```python
from build123d import *

# Parameters (mm, degrees)
SKETCH1_W           = 25.4
SKETCH1_H           = 25.4
BOSS_EXTRUDE1_DEPTH = 63.5
SHELL1_T            = -3.175
SKETCH2_R           = 2.4892
CUT_EXTRUDE1_DEPTH  = 63.5
SKETCH3_R           = 2.53492
CUT_EXTRUDE2_DEPTH  = 63.5


with BuildPart() as part:
    # Sketch1 → Boss-Extrude1 (new body)
    with BuildSketch(Plane.XY):
        with Locations((12.7, 12.7)):
            Rectangle(SKETCH1_W, SKETCH1_H)
    extrude(amount=BOSS_EXTRUDE1_DEPTH)

    # Shell1
    shell1_openings = [part.faces().sort_by_distance(p)[0] for p in [
        (12.7, 12.7, 63.5),
        (12.7, 12.7, 0),
    ]]
    offset(amount=SHELL1_T, openings=shell1_openings, kind=Kind.INTERSECTION)

    # Sketch2 → Cut-Extrude1 (cut)
    with BuildSketch(Plane(origin=(0, 25.4, 0), x_dir=(1, 0, 0), z_dir=(0, 1, 0))):
        with Locations(Location((12.7, -6.35, 0), (0, 0, 270))):
            Circle(SKETCH2_R)
        with Locations(Location((12.7, -19.05, 0), (0, 0, 270))):
            Circle(SKETCH2_R)
        with Locations(Location((12.7, -31.75, 0), (0, 0, 270))):
            Circle(SKETCH2_R)
        with Locations(Location((12.7, -44.45, 0), (0, 0, 270))):
            Circle(SKETCH2_R)
        with Locations(Location((12.7, -57.15, 0), (0, 0, 270))):
            Circle(SKETCH2_R)
    extrude(amount=-CUT_EXTRUDE1_DEPTH, mode=Mode.SUBTRACT)

    # Sketch3 → Cut-Extrude2 (cut)
    with BuildSketch(Plane(origin=(25.4, 0, 0), x_dir=(0, 0, -1), z_dir=(1, 0, 0))):
        with Locations(Location((-57.15, 12.7, 0), (0, 0, 90))):
            Circle(SKETCH3_R)
        with Locations(Location((-44.45, 12.7, 0), (0, 0, 90))):
            Circle(SKETCH3_R)
        with Locations(Location((-31.75, 12.7, 0), (0, 0, 90))):
            Circle(SKETCH3_R)
        with Locations(Location((-19.05, 12.7, 0), (0, 0, 90))):
            Circle(SKETCH3_R)
        with Locations(Location((-6.35, 12.7, 0), (0, 0, 90))):
            Circle(SKETCH3_R)
    extrude(amount=-CUT_EXTRUDE2_DEPTH, mode=Mode.SUBTRACT)


solid = part.part
```
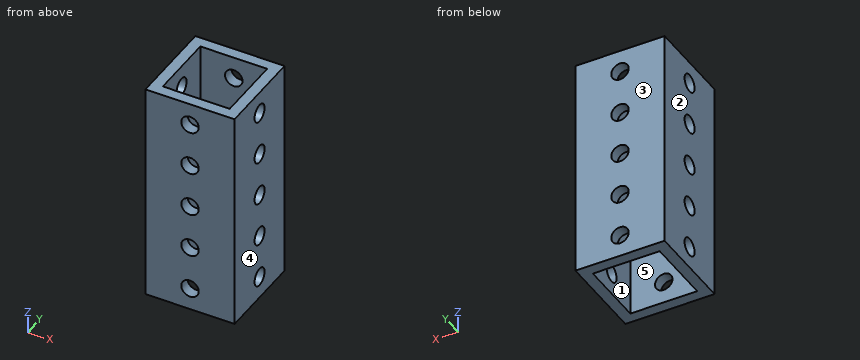
Read the model definition and answer for the solid it produces. Units are mm, in the model's axes. Face numbers are marked on the shaded views. A direction names the side the tool comes from. Give positions to 0.01 mm unless a question says otherwise; leave off trailing zeros. Write each loop counter-clockwise with the first axis right and the second up, starting at its lowest first coordinate (ties: lowest second). Pieces come first, ordered by that corner, then holes. Notation, with made-up numbers: M 0.25,0 L 50.25,0 A28 ccw 50.25,18 Z; hole C -15,-31.5 d9. An arc over 180 degrees is marked long. Put each result on its own line as item: value. Start each with the question number.
1. The part is cut by section B-B, the plane z = 57.15. Give the vertices of the cut face in (x, y) (3 decimals).
2. The part is cut by section A-A, the plane x = 21.5. Give the vertices of the cut face in (y, z) (3 decimals), and give its area (3 significant figures).
3. The part is cut by section D-D, the plane z = 11. Give the vertices of the cut face in (x, y) (3 decimals), and give its area (3 significant figures).
4. Which of the six approach directions +Z, -Z, +X, -X, +Y, -Y give full straight-line access (tool end or side, diameter ignored) to the marked faces 1 and 2?
5. Consider line 1 along Z through (x, y) = (23.05, 12.7); line 2 along X through (y, z) = (7.75, 22) (3 decimals). Determine where each line is inside the solid, lowest interval first.
6. This flat-tipped pin is pushed along its axis until it touches: pin 1 Ø8 at (x, z) = (12.7, 57.15) entering from +Y. Where does it stop, or does it pass through?
7. For a pull along X with two mould halves and no side action, classify the marked faces 3, 4 and 5 as released by +X, released by -X, zero draft, split by the parting line, or undercut.
Final values:
1. outline: M 0,0 L 10.211,0 L 10.211,3.175 L 3.175,3.175 L 3.175,10.165 L 0,10.165 Z; M 0,15.235 L 3.175,15.235 L 3.175,22.225 L 10.211,22.225 L 10.211,25.4 L 0,25.4 Z; M 15.189,0 L 25.4,0 L 25.4,10.165 L 22.225,10.165 L 22.225,3.175 L 15.189,3.175 Z; M 15.189,22.225 L 22.225,22.225 L 22.225,15.235 L 25.4,15.235 L 25.4,25.4 L 15.189,25.4 Z
2. outline: M 0,0 L 3.175,0 L 3.175,63.5 L 0,63.5 Z; M 22.225,0 L 25.4,0 L 25.4,63.5 L 22.225,63.5 Z
2. area: 403 mm²
3. outline: M 0,0 L 25.4,0 L 25.4,25.4 L 0,25.4 Z; hole M 3.175,3.175 L 22.225,3.175 L 22.225,22.225 L 3.175,22.225 Z
3. area: 282 mm²
4. face 1: +Z, -Z
4. face 2: +Z, -Z, -X, +Y, -Y
5. line 1: z = 0 to 3.82, 8.88 to 16.52, 21.58 to 29.22, 34.28 to 41.92, 46.98 to 54.62, 59.68 to 63.5
5. line 2: x = 0 to 3.175, 22.225 to 25.4
6. pin 1: stops at y = 25.4
7. face 3: zero draft
7. face 4: released by +X
7. face 5: undercut
